Could you check a few things on this drawing? It's one solid part, dimensions in mm from its lowest x, y, z. A direction names the side the tool comes from. Give positions to 0.01 mm unless a question says otherwise; leave off trailing zeros. Write each loop counter-clockwise with the first axis right and the second up, starting at its lowest first coordinate (ties: lowest second). Pieces come first, ordered by that corner, then holes. Notation, with made-up numbers: (1.25, 21.25) -> (39.25, 21.25) arc R20 cw to (39.25, 52.25) -> close; hole circle Ø7 at (63, 19). An arc over 180 degrees is marked (long way). Use CSV: the item, a comma, the result in double quotes. Start each with the question number.
(1) For pin 1 Ø1.8 at (x, y) = (28, 28.5) entering from +Z; pin 2 Ø4 at (x, z) = (20.5, 11.5) entering from -Y; pin 3 Ø6.5 at (x, y) = (14, 28.5) entering from +Z, each with a flat end and sliding along its axis, tell me the tip position at first contact or that it passes through.
(2) Which directions (+Z, -Z, +X, -X, +Y, -Y) give clear straight access to the entire face, cutting with the end or side of a thin tool? Please do the marked faces 5, 6 and 7.
(3) If we mould it in two halves opening along X, with no side actions, what happens to the marked faces 1, 2, 3 and 4? For each: pulls with the +X half, pulls with the -X half, needs draft (parallel to the pull), parting line crosses it, or undercut.
(4) Suppose I cut it at B-B on y = 16. List the corners of the cut face in (x, z) for me (1 decimal), plus the area to 3 significant figures.
(5) I need wall thicknesses on L1, parallel to X at y = 6.5, z = 6.25 (1 decimal); L2, parallel to Y at x = 23, z = 21; L3, parallel to Z at x = 18, y = 25. Which ranges of each line are inside material? Lowest first, please. Write a range as [from, to].
(6) Suppose I cut it at A-A on z = 26. List the corners of the cut face in (x, y) for me.
(7) Suppose I cut it at C-C on z = 7.75. List the corners of the cut face in (x, y) for me (1 decimal), plus the area to 3 significant figures.
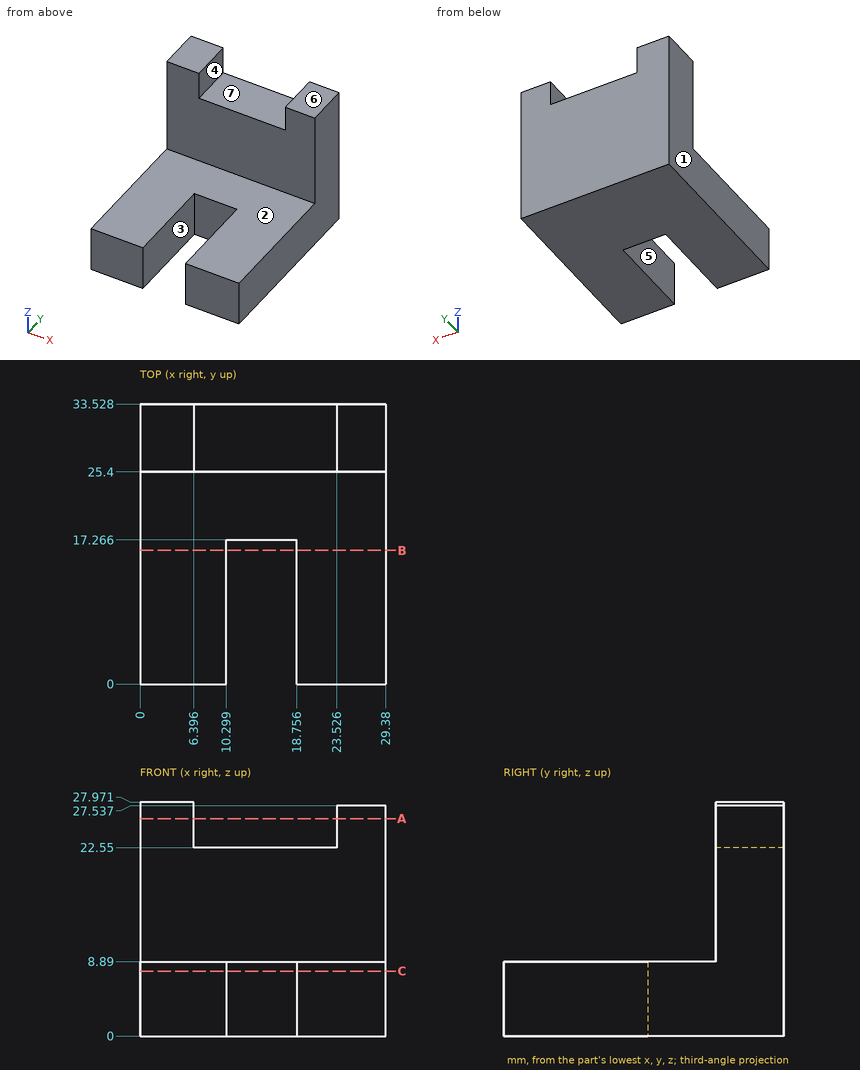
Geometry says:
1,pin 1,"z = 27.54"
1,pin 2,"y = 25.4"
1,pin 3,"z = 22.55"
2,face 5,"+Z, -Z, -Y"
2,face 6,"+Z, +X, +Y, -Y"
2,face 7,"+Z, +Y, -Y"
3,face 1,"pulls with the -X half"
3,face 2,"needs draft"
3,face 3,"undercut"
3,face 4,"undercut"
4,outline,"(0, 0) -> (10.3, 0) -> (10.3, 8.9) -> (0, 8.9) -> close; (18.8, 0) -> (29.4, 0) -> (29.4, 8.9) -> (18.8, 8.9) -> close"
4,area,"186 mm²"
5,L1,"[0, 10.3], [18.8, 29.4]"
5,L2,"[25.4, 33.53]"
5,L3,"[0, 8.89]"
6,outline,"(0, 25.4) -> (6.4, 25.4) -> (6.4, 33.53) -> (0, 33.53) -> close; (23.53, 25.4) -> (29.38, 25.4) -> (29.38, 33.53) -> (23.53, 33.53) -> close"
7,outline,"(0, 0) -> (10.3, 0) -> (10.3, 17.3) -> (18.8, 17.3) -> (18.8, 0) -> (29.4, 0) -> (29.4, 33.5) -> (0, 33.5) -> close"
7,area,"839 mm²"
